```python
from build123d import *

# Parameters (mm, degrees)
F0_W     = 90.17
F0_H     = 91.44
F1_DEPTH = 2.032
F2_SIZE  = 11.43
F3_W     = 68.58
F3_H     = 20.32
F4_DEPTH = 25.4
F5_R     = 1.4605
F6_DEPTH = 6.35


with BuildPart() as f1:
    # F0 (on Top) → F1 (new body)
    with BuildSketch(Plane.XY):
        with Locations((-6.089645, 9.464618)):
            Rectangle(F0_W, F0_H)
    extrude(amount=F1_DEPTH)

    # F2
    f2_edges = [f1.edges().sort_by_distance(p)[0] for p in [
        (-51.174645, 55.184618, 1.016),
        (-51.174645, -36.255382, 1.016),
        (38.995355, 55.184618, 1.016),
        (38.995355, -36.255382, 1.016),
    ]]
    chamfer(f2_edges, length=F2_SIZE)

    # F3 (on Top) → F4 (cut)
    with BuildSketch(Plane.XY):
        with Locations((-6.089645, -27.365382)):
            Rectangle(F3_W, F3_H)
        with Locations((-6.089645, 46.294618)):
            Rectangle(F3_W, F3_H)
    extrude(amount=F4_DEPTH, mode=Mode.SUBTRACT)

    # F5 (on Top) → F6 (join)
    with BuildSketch(Plane.XY):
        with Locations((-26.409645, -14.665382)):
            Circle(F5_R)
        with Locations((25.660355, -9.585382)):
            Circle(F5_R)
        with Locations((25.660355, 18.354618)):
            Circle(F5_R)
        with Locations((-25.139645, 33.594618)):
            Circle(F5_R)
    extrude(amount=F6_DEPTH)


solid = f1.part
```
Source: CAD feature listing. Evaluate the final solid. Frame: model axes, mm. A direction names the side the tool comes from. Round coordinates to 2 decimals unless told otherwise and drop trailing zeros. Loops run counter-clockwise (first coordinate to the right, second up) from the corner with the lowest first, then second, coordinate; pieces in that order, holes last. Notation, with made-up numbers: M -39.5,83.25 L -24.5,83.25 A20 ccw -24.5,92.25 Z; hole C 26.5,58.5 d2. An arc over 180 degrees is marked long. Use a Markdown table: item, result. Add a question column.
1. Cut plane D-D, the plane y = 14. Output: boundary loops of the cut face in (x, z), and give its area (3 significant figures).
2. Cut plane A-A, the plane y = 41. Output: boundary loops of the cut face in (x, z), and give its area (3 significant figures).
3. Contact query for flat-ended pins moving along their axis: pin 1 (1 mm diameter, centred on y = -30, z = 1, fed in from +X); pin 2 (1.6 mm diameter, centred on y = -27.5, z = 0.5, fed in from -X); pin 3 (4 mm diameter, centred on x = 0, y = 30.5, fed in from +Z). Output: stop coordinate, or through.
4. Set-up query: faces 5 (the flat face through (-40.38, -27, 1)), 6 (the flat face through (-45.7, 49.23, 1)), 7 (the cylindrical face through (24.58, -8.6, 4.16)). Return all of +Z, -Z, +X, -X, +Y, -Y with unobstructed straight access to the full face (end or side cutting, diameter ignored); none if empty.
5. Pull-direction query (X, two-part tool) for faces 1 (the flat face through (38.995, 9, 1)), 2 (the cylindrical face through (24.5, 17.47, 4.16)), 3 (the flat face through (26, -10, 6.35)), 4 (the flat face through (-7, 36.135, 1)); classes: +X half, -X half, draft (parallel to the pull), parting line (faces both ways), or undercut.
6. Cut plane C-C, the plane z = 4.75. Output: boundary loops of the cut face in (x, y), and give its area (3 significant figures).
7. Ray query, line 1 along Z through (x, y) = (30, -16.5); line 2 along X through (y, z) = (42, 1.5); line 3 along Y through (x, z) = (14, 1.25). Return the intervals inside material, ascending. Write a range as [from, to].
8. Cut plane B-B, the plane x = 4.5. Output: boundary loops of the cut face in (y, z), and give its area (3 significant figures).
Solution:
| question | item | result |
|---|---|---|
| 1 | outline | M -51.17,0 L 39,0 L 39,2.03 L -51.17,2.03 Z |
| 1 | area | 183 mm2 |
| 2 | outline | M -51.17,0 L -40.38,0 L -40.38,2.03 L -51.17,2.03 Z; M 28.2,0 L 39,0 L 39,2.03 L 28.2,2.03 Z |
| 2 | area | 43.9 mm2 |
| 3 | pin 1 | stops at x = 34.32 |
| 3 | pin 2 | stops at x = -49.3 |
| 3 | pin 3 | stops at z = 2.03 |
| 4 | face 5 | +Z, -Z, -Y |
| 4 | face 6 | +Z, -Z, -X, +Y |
| 4 | face 7 | +Z |
| 5 | face 1 | +X half |
| 5 | face 2 | parting line |
| 5 | face 3 | draft |
| 5 | face 4 | undercut |
| 6 | outline | C -26.41,-14.67 d2.92; C -25.14,33.59 d2.92; C 25.66,-9.59 d2.92; C 25.66,18.35 d2.92 |
| 6 | area | 26.8 mm2 |
| 7 | line 1 | z = [0, 2.03] |
| 7 | line 2 | x = [-51.17, -40.38], [28.2, 39] |
| 7 | line 3 | y = [-17.21, 36.13] |
| 8 | outline | M -17.21,0 L 36.13,0 L 36.13,2.03 L -17.21,2.03 Z |
| 8 | area | 108 mm2 |
